Job drawing, mm, ordinate dimensions from the low corner. One solid piece. A direction names the side the tool comes from. Give positions to 0.01 mm unless a question says otherwise; leave off trailing zeros. Order: outer loops, then holes, each group sorted by start corner. A loop starts at its lowest first (then second) coordinate and runs counter-clockwise, first axis right, second up. Notation, with made-up numbers: (59.25, -9) - (65.25, -9) arc R29 ccw to (65.25, 11) - close; hole circle Ø4 at (-17, 57). An arc over 180 degrees is marked (long way). Use a Markdown table: item, result. Add a question column.
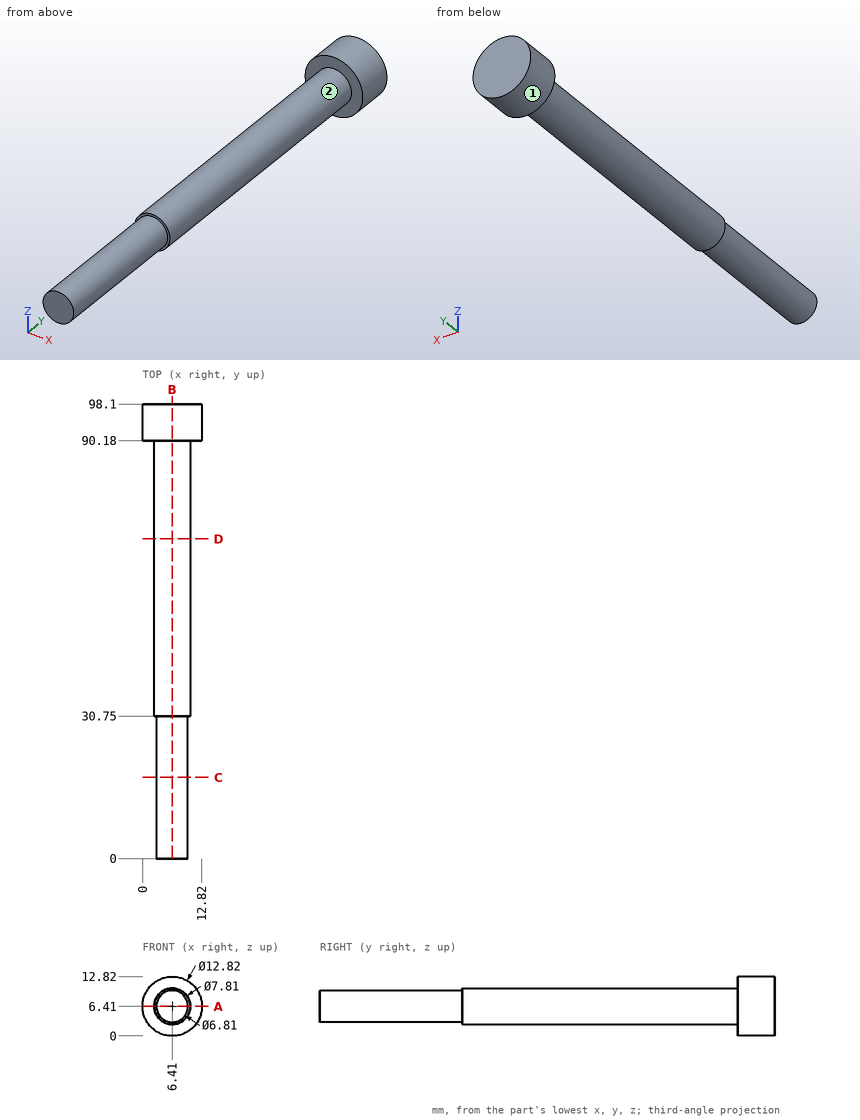
1. Cut at D-D (y = 69). Write the cut outline in (x, z) (3 decimals).
2. Cut at C-C (y = 17.5). Write the cut outline in (x, z) (3 decimals), plus the area to 3 significant figures.
3. Cut at B-B (x = 6.41). Write the cut outline in (y, z) (3 decimals).
4. Tool access for the marked faces 1 and 2: list every direction of +Z, -Z, +X, -X, +Y, -Y with a clear straight run to the whole face (end or side of a thin tool).
5. Cut at A-A (z = 6.41). Write the cut outline in (x, y) (3 decimals), plus the area to 3 significant figures.
6. Drill centre lines: probe 1 along Y at (x, z) = (4, 3.5); probe 2 along Y at (x, z) = (10, 9.25); probe 3 along X at (y, z) = (19, 7.25). Where is each one in solid material? Low to high. Write a range as [from, to].
7. Pin check, flat tips, straight feed: P1, Ø2.5, axis at x = 5.5, z = 8, coming from the -Y side; P2, Ø1, axis at x = 1.5, y = 70, coming from the +Z side; P3, Ø5, axis at x = 2, y = 33.5, coming from the -Z side; P4, Ø5, axis at y = 23.5, z = 8, coming from the +X side (3 decimals). Stop position of each tip, or through.
Responses:
| question | item | result |
|---|---|---|
| 1 | outline | circle Ø7.81 at (6.41, 6.41) |
| 2 | outline | circle Ø6.81 at (6.41, 6.41) |
| 2 | area | 36.4 mm² |
| 3 | outline | (0, 3.005) - (30.75, 3.005) - (30.75, 2.505) - (90.18, 2.505) - (90.18, 0) - (98.1, 0) - (98.1, 12.82) - (90.18, 12.82) - (90.18, 10.315) - (30.75, 10.315) - (30.75, 9.815) - (0, 9.815) - close |
| 4 | face 1 | +Y, -Y |
| 4 | face 2 | -Y |
| 5 | outline | (0, 90.18) - (2.505, 90.18) - (2.505, 30.75) - (3.005, 30.75) - (3.005, 0) - (9.815, 0) - (9.815, 30.75) - (10.315, 30.75) - (10.315, 90.18) - (12.82, 90.18) - (12.82, 98.1) - (0, 98.1) - close |
| 5 | area | 775 mm² |
| 6 | probe 1 | y = [30.75, 98.1] |
| 6 | probe 2 | y = [90.18, 98.1] |
| 6 | probe 3 | x = [3.11, 9.71] |
| 7 | P1 | stops at y = 0 |
| 7 | P2 | passes through |
| 7 | P3 | stops at z = 3 |
| 7 | P4 | stops at x = 9.815 |
